from build123d import *

# Parameters (mm, degrees)
SKETCH_1_W                 = 60
SKETCH_1_H                 = 40
SKETCH_1_W_2               = 56
SKETCH_1_H_2               = 36
EXTRUDE_1_DEPTH            = 92
SKETCH_3_W                 = 21
SKETCH_3_H                 = 24
CUT_EXTRUDE_2_DEPTH        = 41
SKETCH_9_R                 = 3.25
CUT_EXTRUDE_4_DEPTH        = 4
CUT_EXTRUDE_5_REACH        = 62
CUT_EXTRUDE_START          = -55
CUT_EXTRUDE_8_DEPTH        = 30
CUT_EXTRUDE_9_REACH        = 42
SKETCH_17_R                = 5.5
SKETCH_18_W                = 6
SKETCH_18_H                = 1
CUT_EXTRUDE_10_DEPTH       = 61
CUT_EXTRUDE_11_REACH       = 42
HOLE_WIZARD_M31_AT_2_COUNT = 2
HOLE_WIZARD_M31_AT_2_PITCH = 79.506289059
HOLE_WIZARD_M31_AT_3_COUNT = 2
HOLE_WIZARD_M31_AT_3_PITCH = 32.5
CUT_EXTRUDE_12_DEPTH       = 61
CUT_EXTRUDE_13_REACH       = 42


with BuildPart() as part:
    # Эскиз1 → Бобышка-Вытянуть1 (new body)
    with BuildSketch(Plane.XY):
        Rectangle(SKETCH_1_W, SKETCH_1_H)
        Rectangle(SKETCH_1_W_2, SKETCH_1_H_2, mode=Mode.SUBTRACT)
    extrude(amount=EXTRUDE_1_DEPTH)

    # Эскиз3 → Вырез-Вытянуть2 (cut, through all)
    with BuildSketch(Plane(origin=(0, 20, 0), x_dir=(1, 0, 0), z_dir=(0, 1, 0))):
        with Locations((19.5, -60)):
            Rectangle(SKETCH_3_W, SKETCH_3_H)
    extrude(amount=-CUT_EXTRUDE_2_DEPTH, mode=Mode.SUBTRACT)

    # Эскиз9 → Вырез-Вытянуть4 (cut)
    with BuildSketch(Plane.XZ.offset(20)):
        with Locations((21, 11)):
            Circle(SKETCH_9_R)
    extrude(amount=-CUT_EXTRUDE_4_DEPTH, mode=Mode.SUBTRACT)

    # Эскиз10 → Вырез-Вытянуть5 (cut, up to next)
    with BuildSketch(Plane(origin=(30, 0, 0), x_dir=(0, 0, -1), z_dir=(1, 0, 0)), mode=Mode.PRIVATE) as cut_extrude_5_sk1:
        with BuildLine():
            Line((-6, -14.5), (-13, -14.5))
            ThreePointArc((-13, -14.5), (-14.060660172, -14.939339828), (-14.5, -16))
            Line((-14.5, -16), (-14.5, -16.5))
            ThreePointArc((-14.5, -16.5), (-14.060660172, -17.560660172), (-13, -18))
            Line((-13, -18), (-6, -18))
            ThreePointArc((-6, -18), (-4.939339828, -17.560660172), (-4.5, -16.5))
            Line((-4.5, -16.5), (-4.5, -16))
            ThreePointArc((-4.5, -16), (-4.939339828, -14.939339828), (-6, -14.5))
        make_face()
    cut_extrude_5_tool1 = extrude(cut_extrude_5_sk1.sketch, amount=-CUT_EXTRUDE_5_REACH, mode=Mode.PRIVATE) & part.part
    add(cut_extrude_5_tool1.solids().sort_by_distance((30, -16.25, 9.5))[0], mode=Mode.SUBTRACT)

    # Эскиз16 → Вырез-Вытянуть8 (cut)
    with BuildSketch(Plane(origin=(0, 0, 0), x_dir=(-1, 0, 0), z_dir=(0, 0, -1)).offset(CUT_EXTRUDE_START)):
        with BuildLine():
            Line((22.295831523, 20), (12.704168477, 20))
            ThreePointArc((12.704168477, 20), (17.5, 19), (22.295831523, 20))
        make_face()
    extrude(amount=-CUT_EXTRUDE_8_DEPTH, mode=Mode.SUBTRACT)

    # Эскиз17 → Вырез-Вытянуть9 (cut, up to next)
    with BuildSketch(Plane(origin=(0, 20, 0), x_dir=(1, 0, 0), z_dir=(0, 1, 0)), mode=Mode.PRIVATE) as cut_extrude_9_sk1:
        with Locations((19, -16)):
            Circle(SKETCH_17_R)
    cut_extrude_9_tool1 = extrude(cut_extrude_9_sk1.sketch, amount=-CUT_EXTRUDE_9_REACH, mode=Mode.PRIVATE) & part.part
    add(cut_extrude_9_tool1.solids().sort_by_distance((19, 20, 16))[0], mode=Mode.SUBTRACT)

    # Эскиз18 → Вырез-Вытянуть10 (cut, through all)
    with BuildSketch(Plane(origin=(30, 0, 0), x_dir=(0, 0, -1), z_dir=(1, 0, 0))):
        with Locations((-3, -19.5)):
            Rectangle(SKETCH_18_W, SKETCH_18_H)
    extrude(amount=-CUT_EXTRUDE_10_DEPTH, mode=Mode.SUBTRACT)

    # Эскиз19 → Вырез-Вытянуть11 (cut, up to next)
    with BuildSketch(Plane(origin=(0, 20, 0), x_dir=(1, 0, 0), z_dir=(0, 1, 0)), mode=Mode.PRIVATE) as cut_extrude_11_sk1:
        with BuildLine():
            Line((-28, -85.5), (-28, -92))
            Line((-28, -92), (-24.8, -92))
            Line((-24.8, -92), (-24.8, -85.5))
            ThreePointArc((-24.8, -85.5), (-25.239339828, -84.439339828), (-26.3, -84))
            Line((-26.3, -84), (-26.5, -84))
            ThreePointArc((-26.5, -84), (-27.560660172, -84.439339828), (-28, -85.5))
        make_face()
    cut_extrude_11_tool1 = extrude(cut_extrude_11_sk1.sketch, amount=-CUT_EXTRUDE_11_REACH, mode=Mode.PRIVATE) & part.part
    add(cut_extrude_11_tool1.solids().sort_by_distance((-26.4, 20, 88.143673))[0], mode=Mode.SUBTRACT)

    # Эскиз20 → Hole Wizard M31 (revolve, cut)
    with BuildSketch(Plane(origin=(-30, 15.5, 88), x_dir=(0, 0, 1), z_dir=(0, 1, 0))):
        Polygon((0, 0), (0, 2), (1.7, 2), (1.6, 1.9), (1.6, 0.1), (1.7, 0), align=None)
    hole_wizard_m31 = revolve(axis=Axis((-36.35, 15.5, 88), (1, 0, 0)), mode=Mode.SUBTRACT)

    # Hole Wizard M31 at 2: Hole Wizard M31 ×2
    with Locations(*[Vector(0, -0.396195073, -0.91816636) * (i * HOLE_WIZARD_M31_AT_2_PITCH) for i in range(1, HOLE_WIZARD_M31_AT_2_COUNT)]):
        add(hole_wizard_m31, mode=Mode.SUBTRACT)

    # Hole Wizard M31 at 3: Hole Wizard M31 ×2
    with Locations(*[Vector(0, -0.969230769, -0.246153846) * (i * HOLE_WIZARD_M31_AT_3_PITCH) for i in range(1, HOLE_WIZARD_M31_AT_3_COUNT)]):
        add(hole_wizard_m31, mode=Mode.SUBTRACT)

    # Эскиз22 → Вырез-Вытянуть12 (cut, through all)
    with BuildSketch(Plane.ZY.offset(30)):
        Polygon((292.990680401, 5.6), (92, 5.6), (90, 5.6), (90, 4), (92, 4), (292.990680401, 4), (694.972041203, 4), (694.972041203, 5.6), align=None)
    extrude(amount=-CUT_EXTRUDE_12_DEPTH, mode=Mode.SUBTRACT)

    # Эскиз23 → Вырез-Вытянуть13 (cut, up to next)
    with BuildSketch(Plane.XZ.offset(20), mode=Mode.PRIVATE) as cut_extrude_13_sk1:
        with BuildLine():
            Line((-25, 11.5), (-25, 18.5))
            ThreePointArc((-25, 18.5), (-26.5, 20), (-28, 18.5))
            Line((-28, 18.5), (-28, 11.5))
            ThreePointArc((-28, 11.5), (-26.5, 10), (-25, 11.5))
        make_face()
    cut_extrude_13_tool1 = extrude(cut_extrude_13_sk1.sketch, amount=-CUT_EXTRUDE_13_REACH, mode=Mode.PRIVATE) & part.part
    add(cut_extrude_13_tool1.solids().sort_by_distance((-26.5, -20, 15))[0], mode=Mode.SUBTRACT)
    # Эскиз23 → Вырез-Вытянуть13 (cut, up to next)
    with BuildSketch(Plane.XZ.offset(20), mode=Mode.PRIVATE) as cut_extrude_13_sk2:
        with BuildLine():
            Line((-28, 83.5), (-28, 76.5))
            ThreePointArc((-28, 76.5), (-26.5, 75), (-25, 76.5))
            Line((-25, 76.5), (-25, 83.5))
            ThreePointArc((-25, 83.5), (-26.5, 85), (-28, 83.5))
        make_face()
    cut_extrude_13_tool2 = extrude(cut_extrude_13_sk2.sketch, amount=-CUT_EXTRUDE_13_REACH, mode=Mode.PRIVATE) & part.part
    add(cut_extrude_13_tool2.solids().sort_by_distance((-26.5, -20, 80))[0], mode=Mode.SUBTRACT)


solid = part.part
Model file for the job. Use its own axes, mm. A direction names the side the tool comes from. Give positions to 0.01 mm unless a question says otherwise; leave off trailing zeros. Write each loop counter-clockwise with the first axis right and the second up, starting at its lowest first coordinate (ties: lowest second). Pieces come first, ordered by that corner, then holes. Notation, with made-up numbers: (24, 49.25) - (39, 49.25) arc R21 cw to (39, 73.25) - close; hole circle Ø7 at (25.25, 81.5). An arc over 180 degrees is marked (long way). Answer as CSV lines item,"result".
1. Two-plate mould, pull along Y, no slides. Class faces 1 (the face through (0, 18, 45)), 2 (the face through (7, 19, 92)), 3 (the face through (-29.013, -16.481, 16.526)), 4 (the face through (0, -20, 48)): +Y half, -Y half, draft (parallel to the pull), parting line (faces both ways), or undercut.
Responses:
face 1,"undercut"
face 2,"draft"
face 3,"undercut"
face 4,"-Y half"
2. Band-saw the part on A-A (y = 15.5). Write the cut outline in (x, z).
Responses:
outline,"(-30, 0) - (-28, 0) - (-28, 86.3) - (-28.1, 86.4) - (-29.9, 86.4) - (-30, 86.3) - close; (-30, 89.7) - (-29.9, 89.6) - (-28.1, 89.6) - (-28, 89.7) - (-28, 92) - (-30, 92) - close; (28, 0) - (30, 0) - (30, 48) - (28, 48) - close; (28, 72) - (30, 72) - (30, 92) - (28, 92) - close"
3. Band-saw the part on D-D (y = -2.5). Write the cut outline in (x, z), and give its area (3 significant figures).
Responses:
outline,"(-30, 0) - (-28, 0) - (-28, 92) - (-30, 92) - close; (28, 0) - (30, 0) - (30, 48) - (28, 48) - close; (28, 72) - (30, 72) - (30, 92) - (28, 92) - close"
area,"320 mm2"
4. Band-saw the part on B-B (x = -0.5). Write the cut outline in (y, z), and give its area (3 significant figures).
Responses:
outline,"(-20, 6) - (-19, 6) - (-19, 0) - (-18, 0) - (-18, 92) - (-20, 92) - close; (18, 0) - (20, 0) - (20, 92) - (18, 92) - close"
area,"362 mm2"
5. 3-axis set-ups, long thin cutter, end or side, ignore diameter. For faces 5 (the face through (-26.5, -19, 75)), 6 (the face through (28, 0, 24)), 7 (the face through (29, -1, 48)), 8 (the face through (24.08, 19.01, 18.11)): which of +Z, -Z, +X, -X, +Y, -Y reach the whole face in a straight line?
Responses:
face 5,"-Y"
face 6,"+Z, -Z"
face 7,"+X, +Y, -Y"
face 8,"+Y"
6. Pin check, flat tip, straight feed: pin 1 (8 mm diameter, centred on x = 13.5, y = 10.5, fed in from -Z) (1 decimal). Stop position of the tip, or through.
Responses:
pin 1,"passes through"
7. Drill centre lines: L1, parallel to Z at x = 19, y = 19.55; L2, parallel to X at y = -4, z = 40; L3, parallel to Y at x = -29.3, z = 80. Where is each one in solid material? Low to high. Write a range as [from, to].
Responses:
L1,"z = [0, 10.5], [21.5, 48], [72, 92]"
L2,"x = [-30, -28], [28, 30]"
L3,"y = [-20, -17.6], [-14.4, 20]"
8. Band-saw the part on C-C (z = 80). Write the cut outline in (x, y).
Responses:
outline,"(-30, -20) - (-28, -20) - (-28, -17.7) - (-28.1, -17.6) - (-29.9, -17.6) - (-30, -17.7) - close; (-30, -14.3) - (-29.9, -14.4) - (-28.1, -14.4) - (-28, -14.3) - (-28, 18) - (28, 18) - (28, -18) - (-25, -18) - (-25, -20) - (30, -20) - (30, 20) - (-12.7, 20) arc R12 cw to (-22.3, 20) - (-30, 20) - close"
